Could you check a few things on this model? Use its own coordinates, in mm. A direction names the side the tool comes from. Coordinates: 2 decimals unless noted, no trailing zeros. Order: outer loops, then holes, each group sorted by start corner. A loop starts at its lowest first (then second) coordinate and runs counter-clockwise, first axis right, second up. Notation, with made-up numbers: M 75,82 L 119,82 A21 cw 119,114 Z; hole C 4,6.25 d10. An arc over 180 degrees is marked long. Write item = value, one per line. Start each with the question number.
from build123d import *

# Parameters (mm, degrees)
BOSS_EXTRUDE1_DEPTH = 63.5
FILLET1_R           = 31.75
FILLET2_R           = 31.75


with BuildPart() as part:
    # Sketch2 → Boss-Extrude1 (new body, symmetric)
    with BuildSketch(Plane(origin=(0, 0, 0), x_dir=(1, 0, 0), z_dir=(0, 1, 0))):
        Polygon((241.3, -406.4), (241.3, -495.3), (0, -495.3), (0, 495.3), (241.3, 495.3), (241.3, 406.4), (88.9, 406.4), (88.9, -406.4), align=None)
    extrude(amount=BOSS_EXTRUDE1_DEPTH, both=True)

    # Fillet1
    fillet1_edges = [part.edges().sort_by_distance(p)[0] for p in [
        (0, 0, -495.3),
        (0, 0, 495.3),
    ]]
    fillet(fillet1_edges, radius=FILLET1_R)

    # Fillet2
    fillet2_edges = [part.edges().sort_by_distance(p)[0] for p in [
        (0, -63.5, 0),
        (0, 63.5, 0),
        (136.525, 63.5, -495.3),
        (136.525, -63.5, 495.3),
        (9.299359697, -63.5, 486.000640303),
        (9.299359697, -63.5, -486.000640303),
        (136.525, 63.5, 495.3),
        (9.299359697, 63.5, 486.000640303),
        (9.299359697, 63.5, -486.000640303),
        (136.525, -63.5, -495.3),
    ]]
    fillet(fillet2_edges, radius=FILLET2_R)


solid = part.part
(1) Imagine slicing it at D-D on x = 23.5. List the corners of the cut face in (y, z) for me.
(2) Imagine slicing it at A-A on x = 133.5. List the corners of the cut face in (y, z) for me.
(3) Will these pins go through, and if not, where does the flat tip stop? P1, Ø1.5, axis at x = 191.5, y = -42, coming from the +Z side; P2, Ø2, axis at x = 26.5, y = -41.5, coming from the -Z side; P3, Ø3, axis at y = -42.5, z = -303.5, coming from the -X side.
(4) Please list where these lines run through material, in increasing order: probe 1 along Z at (x, y) = (97.5, -3); probe 2 along X at (y, z) = (-28, 398); probe 3 along Z at (x, y) = (158, -55.5). Write a range as from..to.
(5) Imagine slicing it at B-B on y = 15. List the corners of the cut face in (x, z) for me, plus the area to 3 significant figures.
(6) Imagine slicing it at C-C on z = 287.5. List the corners of the cut face in (x, y) for me.
(7) Thinking about a two-plate mould opening in Z: for faces 3 (the cylindrical face through (135.1, -54, 486.2)), 4 (the flat face through (166, 1, -406.4)), 5 (the flat face through (241.3, 1, 450)), 6 (the cylindrical face through (138, 54.4, -485.8)), which applies, released by +Z, released by -Z, zero draft, split by the parting line, or undercut?
(8) For faces 1 (the cylindrical face through (135.1, 54.4, 485.8)), 2 (the flat face through (88.9, 1, -6)), which set-ups out of +Z, -Z, +X, -X, +Y, -Y let a thin tool reach every point of the face, with its end or its side?
Response:
q1.outline = M -62.41,-463.55 A30.66 ccw -31.75,-494.21 L 31.75,-494.21 A30.66 ccw 62.41,-463.55 L 62.41,463.55 A30.66 ccw 31.75,494.21 L -31.75,494.21 A30.66 ccw -62.41,463.55 Z
q2.outline = M -63.5,-463.55 A31.75 ccw -31.75,-495.3 L 31.75,-495.3 A31.75 ccw 63.5,-463.55 L 63.5,-406.4 L -63.5,-406.4 Z; M -63.5,406.4 L 63.5,406.4 L 63.5,463.55 A31.75 ccw 31.75,495.3 L -31.75,495.3 A31.75 ccw -63.5,463.55 Z
q3.P1 = 493.85
q3.P2 = -493.66
q3.P3 = 1.38
q4.probe_1 = -495.3..-406.4, 406.4..495.3
q4.probe_2 = 0..88.9
q4.probe_3 = -484.62..-406.4, 406.4..484.62
q5.outline = M 0,-463.55 A31.75 ccw 31.75,-495.3 L 241.3,-495.3 L 241.3,-406.4 L 88.9,-406.4 L 88.9,406.4 L 241.3,406.4 L 241.3,495.3 L 31.75,495.3 A31.75 ccw 0,463.55 Z
q5.area = 115,000 mm2
q6.outline = M 0,-31.75 A31.75 ccw 31.75,-63.5 L 88.9,-63.5 L 88.9,63.5 L 31.75,63.5 A31.75 ccw 0,31.75 Z
q7.face_3 = released by +Z
q7.face_4 = undercut
q7.face_5 = zero draft
q7.face_6 = released by -Z
q8.face_1 = +Z, +X, -X, +Y
q8.face_2 = +X, +Y, -Y
